Source: CAD feature listing. Evaluate the final solid. Frame: model axes, mm. A direction names the side the tool comes from. Give positions to 0.01 mm unless a question says otherwise; leave off trailing zeros. Loops run counter-clockwise (first coordinate to the right, second up) from the corner with the lowest first, then second, coordinate; pieces in that order, holes last. Notation, with made-up numbers: (17.5, -34) - (28.5, -34) arc R16 ccw to (28.5, -13) - close; hole circle Ø2 at (-2, 59.25). An arc over 180 degrees is marked (long way). Put each result on its own line as item: value.
Autodesk Inventor part; units mm, degrees
ref_plane "YZ Plane" through (0, 0, 0) normal (1, 0, 0) x (0, 1, 0)
ref_plane "XZ Plane" through (0, 0, 0) normal (0, 1, 0) x (-1, 0, 0)
ref_plane "XY Plane" through (0, 0, 0) normal (0, 0, 1) x (1, 0, 0)
sketch "Sketch1" plane through (0, 0, 0) normal (0, 0, 1) x (1, 0, 0)
  point P0 (0, 0)
sketch "Sketch2" plane through (0, 0, 0) normal (0, 0, 1) x (1, 0, 0)
  circle A0 centre (0, 0) radius 32.5
  circle A1 centre (0, 0) radius 19.5
  dimension "d0" = 65
  dimension "d1" = 39
extrude "Extrusion1" add sketch "Sketch2" along normal blind 60
sketch "Sketch3" plane through (0, 0, 60) normal (0, 0, 1) x (1, 0, 0)
  circle A0 centre (0, 0) radius 32.5
extrude "Extrusion2" add sketch "Sketch3" along normal blind 5
sketch "Sketch4" plane through (0, 0, 65) normal (0, 0, 1) x (1, 0, 0)
  circle A0 centre (-15.7, 0) radius 2
  circle A1 centre (0, 0) radius 32.5
  point P0 (2.1, 0)
  dimension "d6" = 4
  dimension "d27" = 15.7
extrude "Extrusion3" cut sketch "Sketch4" against normal blind 5 contours A0
sketch "Sketch5" plane through (0, 0, 65) normal (0, 0, 1) x (1, 0, 0)
  circle A0 centre (0, -7.11) radius 6.5
  point P0 (0, 0)
  dimension "d14" = 7.11
  dimension "d15" = 13
extrude "Extrusion4" cut sketch "Sketch5" against normal blind 5
pattern_circular "Circular Pattern1" count 6 over 360 about axis through (0, 0, -10) along (0, 0, 1) of "Extrusion3"
properties part number "SoporteMotor2"
1) Material intervals for line 1 along Y through (x, z) = (7, 63); line 2 along X through (y, z) = (-0.5, 58); line 3 along X through (y, z) = (15, 45.5), sorted ascending. Write a range as [from, to].
Check result:
line 1: [-31.74, -15.41], [-11.79, 11.79], [15.41, 31.74]
line 2: [-32.5, -19.49], [19.49, 32.5]
line 3: [-28.83, -12.46], [12.46, 28.83]
2) Section query A-A, the plane x = 0. Output: boundary loops of the cut face in (y, z), plus the area to 3 significant figures.
Check result:
outline: (-32.5, 0) - (-19.5, 0) - (-19.5, 60) - (-13.61, 60) - (-13.61, 65) - (-32.5, 65) - close; (-0.61, 60) - (19.5, 60) - (19.5, 0) - (32.5, 0) - (32.5, 65) - (-0.61, 65) - close
area: 1,820 mm²
3) Pin query (flat end, axial travel): P1, Ø5, axis at x = -7.5, z = 28, coming from the +Y side; P2, Ø2.5, axis at x = 15.7, y = 0, coming from the +Z side; P3, Ø12, axis at x = -25, z = 30, coming from the +Y side; P4, Ø1.5, axis at x = 8, z = 38.5, coming from the +Y side. Return the tip coordinate at first contact, or that it passes through.
Check result:
P1: y = 32.11
P2: through
P3: y = 26.37
P4: y = 31.68
4) Section query C-C, the plane x = -7.85. Output: boundary loops of the cut face in (y, z).
Check result:
outline: (-31.54, 0) - (-17.85, 0) - (-17.85, 60) - (-15.6, 60) - (-15.6, 65) - (-31.54, 65) - close; (-11.6, 60) - (11.6, 60) - (11.6, 65) - (-11.6, 65) - close; (15.6, 60) - (17.85, 60) - (17.85, 0) - (31.54, 0) - (31.54, 65) - (15.6, 65) - close
5) Section query D-D, the plane z = 38.5. Output: boundary loops of the cut face in (x, y).
Check result:
outline: circle Ø65 at (0, 0); hole circle Ø39 at (0, 0)
6) Mould query, pull axis X, two halves, no side actions, for faces 3 (the cylindrical face through (-4.791, -2.717, 62.535)), 4 (the flat face through (14, -14, 0)), 5 (the cylindrical face through (31, -9.76, 32.04)). Classes: pulls with the +X half, pulls with the -X half, needs draft (parallel to the pull), parting line crosses it, or undercut.
Check result:
face 3: undercut
face 4: needs draft
face 5: parting line crosses it
7) Section query B-B, the plane y = 13. Output: boundary loops of the cut face in (x, z), plus the area to 3 significant figures.
Check result:
outline: (-29.79, 0) - (-14.53, 0) - (-14.53, 60) - (-9.76, 60) - (-9.76, 65) - (-29.79, 65) - close; (-5.94, 60) - (5.94, 60) - (5.94, 65) - (-5.94, 65) - close; (9.76, 60) - (14.53, 60) - (14.53, 0) - (29.79, 0) - (29.79, 65) - (9.76, 65) - close
area: 2,090 mm²
8) Access query for faces 1 (the cylindrical face through (-6.263, -12.38, 62.535)), 2 (the cylindrical face through (-2.539, -19.334, 29.58)). Directions: +Z, -Z, +X, -X, +Y, -Y. A direction counts if a zero-diameter tool reaches every point of the face in a straight line with its end or side. Return the directions, or none.
Check result:
face 1: +Z, -Z
face 2: -Z
